Source: three-view drawing plus pictorial views. Frame: mm from the lowest corner of the part. A direction names the side the tool comes from. Coordinates: 2 decimals unless noted, no trailing zeros. Write each loop counter-clockwise with the first axis right and the second up, starting at its lowest first coordinate (ties: lowest second). Pieces come first, ordered by that corner, then holes. Notation, with made-up numbers: (56, 13) - (84, 13) arc R16 ccw to (84, 20) - close; hole circle Ø11 at (-4.75, -1.75). An arc over 180 degrees is marked (long way). Put each result on its own line as item: value. Start each with the question number.
1. Line query: line 1 (Y direction, x = 18, z = 2.75); line 2 (Y direction, x = 26.25, z = 1.75); line 3 (X direction, y = 26.25, z = 2). Output: solid intervals per line, ascending.
2. Cut plane D-D, the plane z = 5.75. Return loops of the section in (x, y), and give its area (3 significant figures).
3. Cut plane B-B, the plane z = 2. Return loops of the section in (x, y), and give its area (3 significant figures).
4. Cut plane C-C, the plane y = 26.25. Return loops of the section in (x, z).
5. Cut plane A-A, the plane x = 17.75. Return loops of the section in (y, z).
6. Pin query (flat end, axial travel): pin 1 (3.5 mm diameter, centred on y = 11.5, z = 5, fed in from -X); pin 2 (0.9 mm diameter, centred on x = 10.5, z = 6, fed in from +Y); pin 3 (6.5 mm diameter, centred on x = 17.75, y = 8, fed in from -Z); pin 4 (3.5 mm diameter, centred on x = 11.5, z = 5, fed in from -Y). Return the tip coordinate at first contact, or that it passes through.
7. Pull-direction query (Y, two-part tool) for the marked faces 1, 2 and 3; classes: released by +Y, released by -Y, zero draft, split by the parting line, or undercut.
8. Access query for the marked faces 4, 5 and 6. Directions: +Z, -Z, +X, -X, +Y, -Y. A direction counts if a zero-diameter tool reaches every point of the face in a straight line with its end or side. Return the directions, or none.
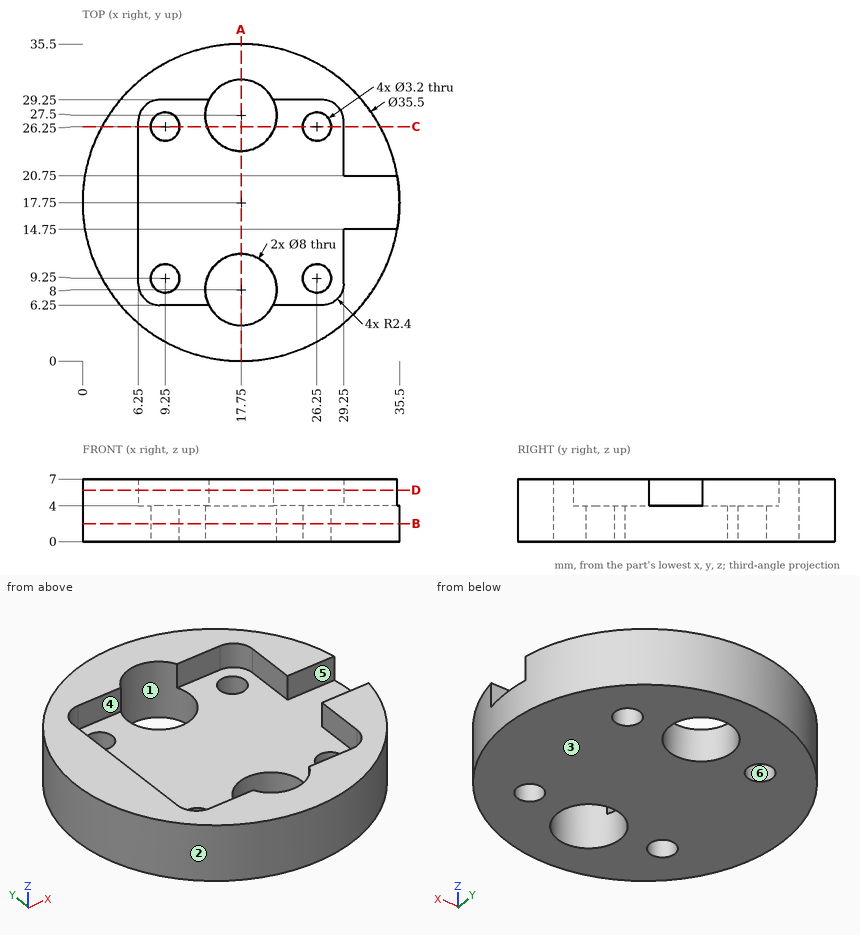
Report:
1. line 1: y = 0 to 4.01, 11.99 to 23.51, 31.49 to 35.5
1. line 2: y = 2.17 to 7.65, 10.85 to 24.65, 27.85 to 33.33
1. line 3: x = 2.17 to 7.65, 10.85 to 13.95, 21.55 to 24.65, 27.85 to 33.33
2. outline: (6.25, 8.65) - (6.25, 26.85) arc R2.4 cw to (8.65, 29.25) - (14.15, 29.25) arc R4 cw to (21.35, 29.25) - (26.85, 29.25) arc R2.4 cw to (29.25, 26.85) - (29.25, 20.75) - (35.24, 20.75) arc R17.75 ccw (long way) to (35.24, 14.75) - (29.25, 14.75) - (29.25, 8.65) arc R2.4 cw to (26.85, 6.25) - (21.35, 6.25) arc R4 cw to (14.15, 6.25) - (8.65, 6.25) arc R2.4 cw to start
2. area: 406 mm^2
3. outline: circle Ø35.5 at (17.75, 17.75); hole circle Ø3.2 at (9.25, 9.25); hole circle Ø3.2 at (9.25, 26.25); hole circle Ø8 at (17.75, 8); hole circle Ø8 at (17.75, 27.5); hole circle Ø3.2 at (26.25, 9.25); hole circle Ø3.2 at (26.25, 26.25)
3. area: 857 mm^2
4. outline: (2.17, 0) - (7.65, 0) - (7.65, 4) - (6.25, 4) - (6.25, 7) - (2.17, 7) - close; (10.85, 0) - (13.95, 0) - (13.95, 4) - (10.85, 4) - close; (21.55, 0) - (24.65, 0) - (24.65, 4) - (21.55, 4) - close; (27.85, 0) - (33.33, 0) - (33.33, 7) - (29.25, 7) - (29.25, 4) - (27.85, 4) - close
5. outline: (0, 0) - (4, 0) - (4, 7) - (0, 7) - close; (12, 0) - (23.5, 0) - (23.5, 4) - (12, 4) - close; (31.5, 0) - (35.5, 0) - (35.5, 7) - (31.5, 7) - close
6. pin 1: stops at x = 0.58
6. pin 2: stops at y = 34.15
6. pin 3: passes through
6. pin 4: stops at y = 0.58
7. face 1: undercut
7. face 2: split by the parting line
7. face 3: zero draft
8. face 4: +Z
8. face 5: +Z, +X
8. face 6: +Z, -Z
